Read the model definition and answer for the solid it produces. Units are mm, in the model's axes. Give positions to 0.01 mm unless a question says otherwise; leave off trailing zeros. Write each loop counter-clockwise with the first axis right and the second up, starting at its lowest first coordinate (ties: lowest second). Pieces come first, ordered by that corner, then holes. Notation, with made-up numbers: M -19,19.25 L 26,19.25 A14 cw 26,26.25 Z; hole C -22,-20.5 d4. An arc over 180 degrees is marked long. Put each result on its own line as item: value.
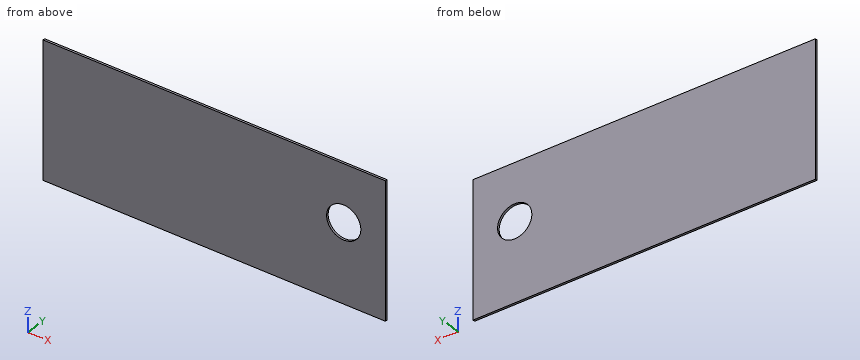
Autodesk Inventor part; units mm, degrees
ref_plane "YZ Plane" through (0, 0, 0) normal (1, 0, 0) x (0, 1, 0)
ref_plane "XZ Plane" through (0, 0, 0) normal (0, 1, 0) x (-1, 0, 0)
ref_plane "XY Plane" through (0, 0, 0) normal (0, 0, 1) x (1, 0, 0)
sketch "Sketch1" plane through (0, 0, 0) normal (0, 1, 0) x (-1, 0, 0)
  line L0 (0, 0) -> (254, 0)
  line L1 (254, 0) -> (254, -101.6)
  line L2 (254, -101.6) -> (0, -101.6)
  line L3 (0, -101.6) -> (0, 0)
  dimension "d0" = 254
  dimension "d1" = 101.6
extrude "Extrusion1" add sketch "Sketch1" along normal blind 1.5875
sketch "Sketch2" plane through (0, 1.5875, 0) normal (0, 1, 0) x (1, 0, 0)
  circle A0 centre (-30.9372, 42.545) radius 12.7
  line L0 (0, 101.6) -> (-254, 101.6)
  line L1 (0, 0) -> (0, 101.6)
  line L2 (-254, 0) -> (0, 0)
  dimension "d4" = 25.4
  dimension "d7" = 30.9372
  dimension "d8" = 42.545
extrude "Extrusion2" cut sketch "Sketch2" against normal blind 25.4
properties part number "TSV+Panel"
(1) Section B-B on z = -33 is taken. Determine the outline of the cut face in (x, y).
Result:
outline: M -254,0 L -39.31,0 L -39.31,1.59 L -254,1.59 Z; M -22.56,0 L 0,0 L 0,1.59 L -22.56,1.59 Z
(2) Section C-C on y = 0.3 is taken. Determine the outline of the cut face in (x, z) (3 decimals), and give its area (3 significant figures).
Result:
outline: M -254,-101.6 L 0,-101.6 L 0,0 L -254,0 Z; hole C -30.937,-42.545 d25.4
area: 25,300 mm²
(3) Given pin 1 Ø1 at (x, z) = (-88.5, -26.5) entering from -Y, flat-ended and moving along its own axis, determine where the tip first touches the part or whether it passes through.
Result:
pin 1: stops at y = 0
(4) Straight lines are drawn through the part: line 1 along X through (y, z) = (1.25, -43.5); line 2 along X through (y, z) = (0.9, -42.5); line 3 along Z through (x, y) = (-25, 0.8). For each, find the intervals that lie inside material, in ascending order. Write a range as from..to.
Result:
line 1: x = -254..-43.6, -18.27..0
line 2: x = -254..-43.64, -18.24..0
line 3: z = -101.6..-53.77, -31.32..0
(5) Section A-A on x = -37 is taken. Determine the outline of the cut face in (y, z).
Result:
outline: M 0,-101.6 L 1.59,-101.6 L 1.59,-53.7 L 0,-53.7 Z; M 0,-31.39 L 1.59,-31.39 L 1.59,0 L 0,0 Z
